from build123d import *

# Parameters (mm, degrees)
F1_DEPTH = 38.1
F2_R     = 12.7
F2_R_2   = 9.525
F3_DEPTH = 6.35


with BuildPart() as f1:
    # F0 (on Right) → F1 (new body)
    with BuildSketch(Plane.YZ):
        Polygon((-31.75, 0), (0, 0), (31.75, 0), (31.75, 12.7), (19.05, 12.7), (19.05, 22.86), (-19.05, 22.86), (-19.05, 12.7), (-31.75, 12.7), align=None)
    extrude(amount=F1_DEPTH)

    # F2 (on face) → F3 (join)
    with BuildSketch(Plane.XY.offset(22.86)):
        with Locations((19.05, 0)):
            Circle(F2_R)
        with Locations((19.05, 0)):
            Circle(F2_R_2, mode=Mode.SUBTRACT)
    extrude(amount=F3_DEPTH)


solid = f1.part
Verification items for the finished model (mm, model axes). A direction names the side the tool comes from. Give positions to 0.01 mm unless a question says otherwise; leave off trailing zeros. Write each loop counter-clockwise with the first axis right and the second up, starting at its lowest first coordinate (ties: lowest second). Pieces come first, ordered by that corner, then holes. Notation, with made-up numbers: M 88,7.5 L 98,7.5 A13 cw 98,27.5 Z; hole C 13,-24.75 d9. An arc over 180 degrees is marked long. Write item = value, one per line.
(1) Draft check along Y on faces 1 (the face through (19, -31.75, 6)), 2 (the face through (19, 0, 22.86)), 3 (the face through (19, -25, 12.7)). Enter one of: released by +Y, released by -Y, zero draft, split by the parting line, or undercut.
Found:
face_1 = released by -Y
face_2 = undercut
face_3 = zero draft
(2) Sectioned sample at C-C (z = 27.25). Record the cut outline in (x, y) (3 decimals).
Found:
outline = C 19.05,0 d25.4; hole C 19.05,0 d19.05
(3) Go/stop test with flat-tipped pins: pin 1 Ø4 at (x, y) = (17, 28) entering from +Z; pin 2 Ø8 at (x, y) = (21, -2) entering from +Z; pin 3 Ø5 at (x, z) = (15, 19.5) entering from +Y. Record where each tip stops, or that it passes through.
Found:
pin_1 = 12.7
pin_2 = 22.86
pin_3 = 19.05
(4) Sectioned sample at B-B (y = 0). Record the cut outline in (x, z) (3 decimals).
Found:
outline = M 0,0 L 38.1,0 L 38.1,22.86 L 31.75,22.86 L 31.75,29.21 L 28.575,29.21 L 28.575,22.86 L 9.525,22.86 L 9.525,29.21 L 6.35,29.21 L 6.35,22.86 L 0,22.86 Z
(5) Access from +Z, -Z, +X, -X, +Y, -Y to the whole of each face (thin tool, end or side, straight path). Record for faces 4 (the face through (19, -19.05, 18)), 5 (the face through (31.164, 3.815, 25.991)), 6 (the face through (38.1, 0, 9)), 7 (the face through (19, 25, 12.7)).
Found:
face_4 = +Z, +X, -X, -Y
face_5 = +Z
face_6 = +Z, -Z, +X, +Y, -Y
face_7 = +Z, +X, -X, +Y
(6) Sectioned sample at A-A (x = 4.5). Record the cut outline in (y, z).
Found:
outline = M -31.75,0 L 31.75,0 L 31.75,12.7 L 19.05,12.7 L 19.05,22.86 L -19.05,22.86 L -19.05,12.7 L -31.75,12.7 Z
(7) Material ranges on line 1 (Y direction, x = 19.05, z = 24.75) (3 decimals); line 2 (Z direction, x = 28.5, y = -12.5); line 3 (Z direction, x = 19, y = 27.5), recorded low to high.
Found:
line_1 = -12.7 to -9.525, 9.525 to 12.7
line_2 = 0 to 22.86
line_3 = 0 to 12.7
(8) Sectioned sample at D-D (x = 19.05). Record the cut outline in (y, z) (3 decimals).
Found:
outline = M -31.75,0 L 31.75,0 L 31.75,12.7 L 19.05,12.7 L 19.05,22.86 L 12.7,22.86 L 12.7,29.21 L 9.525,29.21 L 9.525,22.86 L -9.525,22.86 L -9.525,29.21 L -12.7,29.21 L -12.7,22.86 L -19.05,22.86 L -19.05,12.7 L -31.75,12.7 Z
